Check sheet for the modelled part. Datum: model origin and axes. Units: mm. Face numbers are marked on the shaded views. A direction names the side the tool comes from. Give positions to 0.01 mm unless a question says otherwise; leave off trailing zeros. Write each loop counter-clockwise with the first axis right and the second up, starting at its lowest first coordinate (ties: lowest second). Pieces come first, ordered by that corner, then holes. Notation, with made-up numbers: (70.5, -38) -> (112.5, -38) arc R20 ccw to (112.5, -19) -> close; hole circle Ø6 at (-17, 66). An arc over 180 degrees is marked (long way). Return JSON: item names as keys, results as strings.
Autodesk Inventor part; units mm, degrees
ref_plane "YZ Plane" through (0, 0, 0) normal (1, 0, 0) x (0, 1, 0)
ref_plane "XZ Plane" through (0, 0, 0) normal (0, 1, 0) x (-1, 0, 0)
ref_plane "XY Plane" through (0, 0, 0) normal (0, 0, 1) x (1, 0, 0)
sketch "Sketch1" plane through (0, 0, 0) normal (0, 1, 0) x (-1, 0, 0)
  circle A0 centre (0, 0) radius 1.5
  dimension "d0" = 3
extrude "Extrusion1" add sketch "Sketch1" along normal blind 2.5
sketch "Sketch2" plane through (0, 2.5, 0) normal (0, 1, 0) x (1, 0, 0)
  circle A0 centre (0, 0) radius 2
  dimension "d3" = 4
extrude "Extrusion2" add sketch "Sketch2" along normal blind 8.5
thread "Thread1"
sketch "Sketch3" plane through (0, 11, 0) normal (0, 1, 0) x (1, 0, 0)
  circle A0 centre (0, 0) radius 2
  dimension "d8" = 4
extrude "Extrusion3" add sketch "Sketch3" along normal blind 1 draft -60
sketch "Sketch4" plane through (0, 12, 0) normal (0, 1, 0) x (1, 0, 0)
  line L0 (-0.15, 1.5) -> (0.15, 1.5)
  line L1 (0.2, 1.45) -> (0.2, 0.25)
  line L2 (0.15, -1.5) -> (-0.15, -1.5)
  line L3 (-0.2, 0.25) -> (-0.2, 1.45)
  line L4 (-0.2, 1.5) -> (0.2, -1.5) construction
  line L5 (0.2, 1.5) -> (-0.2, -1.5) construction
  line L6 (0.25, 0.2) -> (1.45, 0.2)
  line L7 (1.5, 0.15) -> (1.5, -0.15)
  line L8 (1.45, -0.2) -> (0.25, -0.2)
  line L9 (-1.5, -0.15) -> (-1.5, 0.15)
  circle A0 centre (0, 0) radius 0.2679
  line L10 (-1.5, 0.2) -> (1.5, -0.2) construction
  line L11 (1.5, 0.2) -> (-1.5, -0.2) construction
  arc A1 (-0.15, 1.5) -> (-0.2, 1.45) centre (-0.15, 1.45) ccw
  arc A2 (0.2, 1.45) -> (0.15, 1.5) centre (0.15, 1.45) ccw
  arc A3 (0.2, 0.25) -> (0.25, 0.2) centre (0.25, 0.25) ccw
  arc A4 (1.5, 0.15) -> (1.45, 0.2) centre (1.45, 0.15) ccw
  arc A5 (1.45, -0.2) -> (1.5, -0.15) centre (1.45, -0.15) ccw
  line L12 (0.2, -1.45) -> (0.2, -0.25)
  line L13 (-1.45, 0.2) -> (-0.25, 0.2)
  arc A6 (0.25, -0.2) -> (0.2, -0.25) centre (0.25, -0.25) ccw
  arc A7 (-0.25, 0.2) -> (-0.2, 0.25) centre (-0.25, 0.25) ccw
  line L14 (-1.45, -0.2) -> (-0.25, -0.2)
  line L15 (-0.2, -1.45) -> (-0.2, -0.25)
  arc A8 (-0.2, -0.25) -> (-0.25, -0.2) centre (-0.25, -0.25) ccw
  arc A9 (-1.45, 0.2) -> (-1.5, 0.15) centre (-1.45, 0.15) ccw
  arc A10 (-1.5, -0.15) -> (-1.45, -0.2) centre (-1.45, -0.15) ccw
  arc A11 (-0.2, -1.45) -> (-0.15, -1.5) centre (-0.15, -1.45) ccw
  arc A12 (0.15, -1.5) -> (0.2, -1.45) centre (0.15, -1.45) ccw
  point P0 (0.25, 0.2)
  point P1 (0.3698, -0.2)
  point P2 (-0.2, 0.3871)
  dimension "d11" = 0.4
  dimension "d12" = 3
  dimension "d13" = 3
  dimension "d14" = 0.4
  dimension "d15" = 0.05
  dimension "d16" = 0.05
  dimension "d17" = 0.05
extrude "Extrusion4" cut sketch "Sketch4" against normal blind 1 contours L0 A2 L1 A3 L6 A4 L7 A5 L8 A6 L12 A12 L2 A11 L15 A8 L14 A10 L9 A9 L13 A7 L3 A1 | A0
properties material "Stainless Steel"
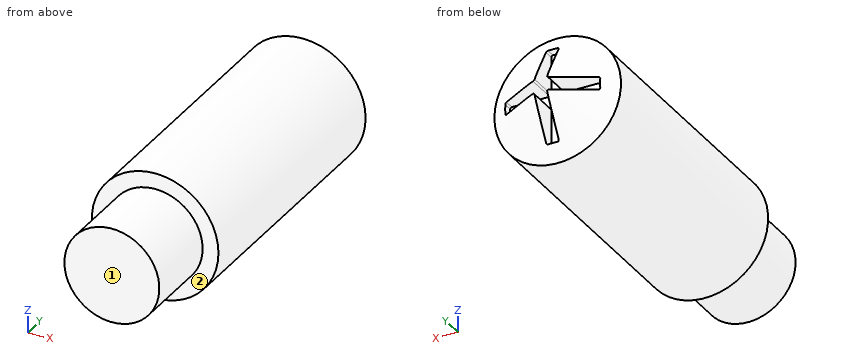
(1) Depth check by flat-ended pin: pin 1 Ø1.2 at (x, z) = (0.5, -0.5) entering from -Y; pin 2 Ø0.5 at (y, z) = (11.5, 1) entering from +X; pin 3 Ø2 at (x, z) = (-1, -1) entering from +Y; pin 4 Ø0.8 at (x, y) = (1, 11.5) entering from -Z. Enter the tip coordinate at first touch or a pass-through.
Reply:
{"pin 1": "y = 0", "pin 2": "x = 1.24", "pin 3": "y = 11.92", "pin 4": "z = -1.56"}
(2) Set-up check for the marked faces 1 and 2: record each of +Z, -Z, +X, -X, +Y, -Y from which the full face is reachable in a straight line by a thin tool's end or side.
Reply:
{"face 1": "+Z, -Z, +X, -X, -Y", "face 2": "-Y"}
(3) Cross-section at A-A on x = 0. Enter the section's corners in (y, z).
Reply:
{"outline": "(0, -1.5) -> (2.5, -1.5) -> (2.5, -2) -> (11, -2) -> (11.29, -1.5) -> (11, -1.5) -> (11, 1.5) -> (11.29, 1.5) -> (11, 2) -> (2.5, 2) -> (2.5, 1.5) -> (0, 1.5) -> close"}
(4) Thickness scan on L1, parallel to Y at x = -0.05, z = 0.65; L2, parallel to X at y = 8.75, z = -0.55; L3, parallel to Y at x = 0.95, z = 0.35. Record the ranges inside material, lowest first.
Reply:
{"L1": "0 to 11", "L2": "-1.92 to 1.92", "L3": "0 to 11.57"}
(5) Cross-section at B-B on z = 0. Enter the section's corners in (x, y), then the cut area to 3 significant figures.
Reply:
{"outline": "(-2, 2.5) -> (-1.5, 2.5) -> (-1.5, 0) -> (1.5, 0) -> (1.5, 2.5) -> (2, 2.5) -> (2, 11) -> (1.5, 11.29) -> (1.5, 11) -> (-1.5, 11) -> (-1.5, 11.29) -> (-2, 11) -> close", "area": "41.6 mm^2"}
(6) Cross-section at C-C on y = 4.75. Enter the section's corners in (x, z).
Reply:
{"outline": "circle Ø4 at (0, 0)"}
